Build history of the part. All positions in model axes, mm. A direction names the side the tool comes from. Round coordinates to 2 decimals unless told otherwise and drop trailing zeros. Write each loop counter-clockwise with the first axis right and the second up, starting at its lowest first coordinate (ties: lowest second). Pieces come first, ordered by that corner, then holes.
from build123d import *

# Parameters (mm, degrees)
BOSS_EXTRUDE1_DEPTH     = 20
CUT_EXTRUDE1_START      = -20
CUT_EXTRUDE1_DEPTH      = 20
SKETCH4_R               = 1.9
BOSS_EXTRUDE2_DEPTH     = 3
BOSS_EXTRUDE3_DEPTH     = 2
INTERSECT3_START        = -3.545087111
INTERSECT3_DEPTH        = 2
CUT_EXTRUDE3_DEPTH      = 12
CUT_EXTRUDE3_DEPTH_BACK = 42.091890171
SKETCH9_R               = 1.75
BOSS_EXTRUDE4_START     = 2
SKETCH10_R              = 2.75
SKETCH10_R_2            = 1.75
BOSS_EXTRUDE4_DEPTH     = 2


with BuildPart() as part:
    # Sketch1 → Boss-Extrude1 (new body)
    with BuildSketch(Plane(origin=(0, 0, -0.380808332), x_dir=(-1, 0, 0), z_dir=(0, 0, -1))):
        with BuildLine():
            Line((7.571744633, 37.567534319), (2.583293076, 37.567534319))
            ThreePointArc((2.583293076, 37.567534319), (-7.416706924, 27.567534319), (2.583293076, 17.567534319))
            Line((2.583293076, 17.567534319), (7.571744633, 17.567534319))
            Line((7.571744633, 17.567534319), (7.571744633, 19.567534319))
            Line((7.571744633, 19.567534319), (-0.416706924, 19.567534319))
            Line((-0.416706924, 19.567534319), (-0.416706924, 35.567534319))
            Line((-0.416706924, 35.567534319), (7.571744633, 35.567534319))
            Line((7.571744633, 35.567534319), (7.571744633, 37.567534319))
        make_face()
    extrude(amount=BOSS_EXTRUDE1_DEPTH)

    # Cut-Extrude1: read off the stored shape, not the designer's step
    # Cut-Extrude1 outline → Cut-Extrude1 (cut)
    with BuildSketch(Plane.XZ.offset(-17.567534319).offset(CUT_EXTRUDE1_START)):
        Polygon((-7.571744633, -0.380808332), (-7.571744633, -20.380808332), (7.416706924, -20.380808332), (7.416706924, -7.370038076), align=None)
    extrude(amount=CUT_EXTRUDE1_DEPTH, mode=Mode.SUBTRACT)

    # Sketch4 → Boss-Extrude2 (add)
    with BuildSketch(Plane.XY.offset(-0.380808332)):
        with Locations(Location((3.916706924, 30.067534319, 0), (0, 0, 180))):
            Circle(SKETCH4_R)
        with Locations(Location((3.916706924, 25.067534319, 0), (0, 0, 180))):
            Circle(SKETCH4_R)
    extrude(amount=BOSS_EXTRUDE2_DEPTH)



with BuildPart() as body_2:
    # Sketch5 → Boss-Extrude3 (new body)
    with BuildSketch(Plane(origin=(-1.498218553, 0, -3.212940055), x_dir=(-0.9063077870366496, 0, 0.42261826174070033), z_dir=(-0.4226182617407003, 0, -0.9063077870366495))):
        with BuildLine():
            Line((-5.80275273, 35.29745693), (-5.80275273, 37.567534319))
            ThreePointArc((-5.80275273, 37.567534319), (-15.80275273, 27.567534319), (-5.80275273, 17.567534319))
            Line((-5.80275273, 17.567534319), (-5.80275273, 19.837611709))
            add(Edge.make_bspline(
                [(-5.80275273, 35.29745693), (-9.83653192, 32.297006625), (-9.83653192, 27.567534319), (-9.83653192, 22.838062014), (-5.80275273, 19.837611709)],
                knots=[2.263071394, 2.263071394, 2.263071394, 3.141592654, 3.141592654, 4.020113913, 4.020113913, 4.020113913], degree=2, weights=[0.855612192, 0.836189508, 1, 0.836189508, 0.855612192]))
        make_face()
        with BuildLine():
            Line((-5.80275273, 19.837611709), (-5.80275273, 17.567534319))
            Line((-5.80275273, 17.567534319), (1.19724727, 17.567534319))
            add(Edge.make_bspline(
                [(-5.80275273, 19.837611709), (-2.750880511, 17.567534319), (1.19724727, 17.567534319)],
                knots=[4.020113913, 4.020113913, 4.020113913, 4.71238898, 4.71238898, 4.71238898], degree=2, weights=[0.855612192, 0.870917273, 1]))
        make_face()
        with BuildLine():
            Line((1.19724727, 37.567534319), (-5.80275273, 37.567534319))
            Line((-5.80275273, 37.567534319), (-5.80275273, 35.29745693))
            add(Edge.make_bspline(
                [(1.19724727, 37.567534319), (-2.750880511, 37.567534319), (-5.80275273, 35.29745693)],
                knots=[1.570796327, 1.570796327, 1.570796327, 2.263071394, 2.263071394, 2.263071394], degree=2, weights=[1, 0.870917273, 0.855612192]))
        make_face()
    extrude(amount=-BOSS_EXTRUDE3_DEPTH)


with BuildPart() as part_1:
    add(part.part)

    add(body_2.part)  # Intersect3 merges body 2
    # Intersect3: read off the stored shape, not the designer's step
    # Intersect3 outline → Intersect3 (add)
    with BuildSketch(Plane(origin=(0, 0, 0), x_dir=(0.9063077870366488, 0, -0.42261826174070194), z_dir=(0.4226182617407019, 0, 0.9063077870366488)).offset(INTERSECT3_START)):
        with BuildLine():
            ThreePointArc((5.80275273, 17.567534319), (15.80275273, 27.567534319), (5.80275273, 37.567534319))
            Line((5.80275273, 37.567534319), (-2.129862586, 37.567534319))
            add(Edge.make_bspline(
                [(-2.129862586, 17.567534319), (8.903916604, 17.567534319), (8.903916604, 27.567534319), (8.903916604, 37.567534319), (-2.129862586, 37.567534319)],
                knots=[1.570796327, 1.570796327, 1.570796327, 3.141592654, 3.141592654, 4.71238898, 4.71238898, 4.71238898], degree=2, weights=[1, 0.707106781, 1, 0.707106781, 1]))
            Line((-2.129862586, 17.567534319), (5.80275273, 17.567534319))
        make_face()
    extrude(amount=INTERSECT3_DEPTH)

    # Sketch9 → Cut-Extrude3 (cut, two sides: drawn at the far end of the back side and taken through both)
    with BuildSketch(Plane(origin=(-0.652982029, 0, -1.400324481), x_dir=(0.9063077870366496, 0, -0.4226182617407002), z_dir=(0.4226182617407003, 0, 0.9063077870366497)).offset(-CUT_EXTRUDE3_DEPTH_BACK)):
        with Locations(Location((12.353334667, 27.567534319, 0), (0, 0, 180))):
            Circle(SKETCH9_R)
    extrude(amount=CUT_EXTRUDE3_DEPTH + CUT_EXTRUDE3_DEPTH_BACK, mode=Mode.SUBTRACT)

    # Sketch10 → Boss-Extrude4 (add)
    with BuildSketch(Plane(origin=(-0.652982029, 0, -1.400324481), x_dir=(0.9063077870366488, 0, -0.4226182617407019), z_dir=(0.4226182617407019, 0, 0.9063077870366488)).offset(BOSS_EXTRUDE4_START)):
        with Locations((12.353334667, 27.567534319)):
            Circle(SKETCH10_R)
        with Locations(Location((12.353334667, 27.567534319, 0), (0, 0, 180))):
            Circle(SKETCH10_R_2, mode=Mode.SUBTRACT)
    extrude(amount=-BOSS_EXTRUDE4_DEPTH)


solid = part_1.part
1) Wall check: L1, parallel to Y at x = -6.25, z = -0.75; L2, parallel to Y at x = 11.5, z = -5.5; L3, parallel to X at y = 23, z = -6. Give the ranges that are in metal, low to high.
Results:
L1: y = 17.57 to 19.57, 35.57 to 37.57
L2: y = 24.85 to 25.86, 29.27 to 30.29
L3: x = 4.48 to 9.21
2) Mould opens along Z. For faces 1 (the flat face through (-2, 19.568, -1)), 2 (the cylindrical face through (13.238, 27.787, -8.997)), 3 (the cylindrical face through (10.647, 30.294, -5.551)) say: released by +Z, released by -Z, zero draft, split by the parting line, or undercut.
Results:
face 1: zero draft
face 2: released by -Z
face 3: undercut
3) Slice it at D-D (z = -3.25). Write the cut outline in (x, y), plus the area to 3 significant figures.
Results:
outline: (-1.42, 17.57) - (3.31, 17.57) - (3.31, 19.49) arc R10 ccw to (3.31, 35.64) - (3.31, 37.57) - (-1.42, 37.57) - (-1.42, 35.57) - (0.42, 35.57) - (0.42, 19.57) - (-1.42, 19.57) - close
area: 112 mm2
4) Slice it at C-C (y = 21.5). Write the cut outline in (x, z), plus the area to 3 significant figures.
Results:
outline: (0.42, -4.11) - (10.97, -9.02) - (11.81, -7.21) - (5.37, -4.21) - (5.37, -0.38) - (0.42, -0.38) - close
area: 37.4 mm2
5) Pin check, flat tips, straight feed: pin 1 Ø1.9 at (y, z) = (31.5, -2) entering from -X; pin 2 Ø4.5 at (x, y) = (-1.5, 26) entering from +Z; pin 3 Ø1.5 at (y, z) = (25, -4) entering from +X; pin 4 Ø1 at (x, y) = (-0.5, 23.5) entering from -Z. Stop position of each tip, or through.
Results:
pin 1: stops at x = 0.42
pin 2: stops at z = -0.38
pin 3: stops at x = 11.26
pin 4: passes through
6) Slice it at B-B (x = 1.75). Write the cut outline in (y, z), plus the area to 3 significant figures.
Results:
outline: (17.57, -4.73) - (37.57, -4.73) - (37.57, -2.52) - (36.58, -2.52) - (36.58, -0.38) - (18.56, -0.38) - (18.56, -2.52) - (17.57, -2.52) - close
area: 82.7 mm2
7) Slice it at A-A (x = -4.5). Write the cut outline in (y, z).
Results:
outline: (17.57, -1.81) - (19.57, -1.81) - (19.57, -0.38) - (17.57, -0.38) - close; (35.57, -1.81) - (37.57, -1.81) - (37.57, -0.38) - (35.57, -0.38) - close
8) Which spindle directions (+Z, -Z, +X, -X, +Y, -Y) get a long thin tool onto all of the face, cutting with end or side? Do faces 4 (the flat face through (0, 17.568, -3)), 5 (the flat face through (-3, 35.568, -2)), 6 (the cylindrical face through (3.04, 31.753, 1.098)). Say none if no direction does.
Results:
face 4: +Z, -Z, +X, -X, -Y
face 5: +Z, -Z, -X
face 6: +Z
